Geometry check sheet. Reference: the model listing, model coordinates, mm. A direction names the side the tool comes from. Round coordinates to 2 decimals unless told otherwise and drop trailing zeros. Order: outer loops, then holes, each group sorted by start corner. A loop starts at its lowest first (then second) coordinate and runs counter-clockwise, first axis right, second up. Notation, with made-up numbers: (72, 39) -> (102, 39) arc R27 ccw to (102, 56) -> close; hole circle Ø8 at (86, -27.75). An arc over 180 degrees is marked (long way). Use a Markdown table: item, result. Add a question column.
Item 1: Set-up check for faces 1 (the flat face through (7.875, -18, 1)), 2 (the flat face through (18, -3, 1)), 3 (the flat face through (0, -3, 1)): record each of +Z, -Z, +X, -X, +Y, -Y from which the full face is reachable in a straight line by a thin tool's end or side.
Item 2: Sectioned sample at C-C, the plane x = -3.5. Record the cut outline in (y, z).
Item 3: Sectioned sample at B-B, the plane y = -17. Record the cut outline in (x, z) (3 decimals).
Item 4: Material ranges on probe 1 along X at (y, z) = (-28, 0.75) (3 decimals); probe 2 along Y at (x, z) = (-5, 0.9), recorded low to high. Write a range as [from, to].
Item 5: Sectioned sample at A-A, the plane z = 0.75. Record the cut outline in (x, y) (3 decimals), and give its area (3 significant figures).
Item 6: Gauge pin test, flat end, axial feed: pin 1 Ø0.8 at (y, z) = (-15, 0.5) entering from +X. Record the tip position at first contact, or that the pin passes through.
from build123d import *

# Parameters (mm, degrees)
F1_DEPTH = 1.5


with BuildPart() as f1:
    # F0 (on Top) → F1 (new body)
    with BuildSketch(Plane.XY):
        with BuildLine():
            Line((22.5, 0), (-22.5, 0))
            Line((-22.5, 0), (-22.5, -3))
            Line((-22.5, -3), (-13.5, -3))
            Line((-13.5, -3), (-13.5, -33.25))
            ThreePointArc((-13.5, -33.25), (-13.06066, -34.31066), (-12, -34.75))
            Line((-12, -34.75), (-6.75, -34.75))
            ThreePointArc((-6.75, -34.75), (-5.68934, -34.31066), (-5.25, -33.25))
            Line((-5.25, -33.25), (-5.25, -3))
            Line((-5.25, -3), (5.25, -3))
            Line((5.25, -3), (5.25, -33.25))
            ThreePointArc((5.25, -33.25), (5.68934, -34.31066), (6.75, -34.75))
            Line((6.75, -34.75), (12, -34.75))
            ThreePointArc((12, -34.75), (13.06066, -34.31066), (13.5, -33.25))
            Line((13.5, -33.25), (13.5, -3))
            Line((13.5, -3), (22.5, -3))
            Line((22.5, -3), (22.5, 0))
        make_face()
        with BuildLine():
            ThreePointArc((-10.875, -4.5), (-9.375, -3), (-7.875, -4.5))
            Line((-7.875, -4.5), (-7.875, -30.25))
            ThreePointArc((-7.875, -30.25), (-9.375, -31.75), (-10.875, -30.25))
            Line((-10.875, -30.25), (-10.875, -4.5))
        make_face(mode=Mode.SUBTRACT)
        with BuildLine():
            ThreePointArc((7.875, -4.5), (9.375, -3), (10.875, -4.5))
            Line((10.875, -4.5), (10.875, -30.25))
            ThreePointArc((10.875, -30.25), (9.375, -31.75), (7.875, -30.25))
            Line((7.875, -30.25), (7.875, -4.5))
        make_face(mode=Mode.SUBTRACT)
    extrude(amount=F1_DEPTH)


solid = f1.part
Found:
| question | item | result |
|---|---|---|
| 1 | face 1 | +Z, -Z |
| 1 | face 2 | +Z, -Z, +X, -Y |
| 1 | face 3 | +Z, -Z, -Y |
| 2 | outline | (-3, 0) -> (0, 0) -> (0, 1.5) -> (-3, 1.5) -> close |
| 3 | outline | (-13.5, 0) -> (-10.875, 0) -> (-10.875, 1.5) -> (-13.5, 1.5) -> close; (-7.875, 0) -> (-5.25, 0) -> (-5.25, 1.5) -> (-7.875, 1.5) -> close; (5.25, 0) -> (7.875, 0) -> (7.875, 1.5) -> (5.25, 1.5) -> close; (10.875, 0) -> (13.5, 0) -> (13.5, 1.5) -> (10.875, 1.5) -> close |
| 4 | probe 1 | x = [-13.5, -10.875], [-7.875, -5.25], [5.25, 7.875], [10.875, 13.5] |
| 4 | probe 2 | y = [-3, 0] |
| 5 | outline | (-22.5, -3) -> (-13.5, -3) -> (-13.5, -33.25) arc R1.5 ccw to (-12, -34.75) -> (-6.75, -34.75) arc R1.5 ccw to (-5.25, -33.25) -> (-5.25, -3) -> (5.25, -3) -> (5.25, -33.25) arc R1.5 ccw to (6.75, -34.75) -> (12, -34.75) arc R1.5 ccw to (13.5, -33.25) -> (13.5, -3) -> (22.5, -3) -> (22.5, 0) -> (-22.5, 0) -> close; hole (-10.875, -30.25) arc R1.5 ccw to (-7.875, -30.25) -> (-7.875, -4.5) arc R1.5 ccw to (-10.875, -4.5) -> close; hole (7.875, -30.25) arc R1.5 ccw to (10.875, -30.25) -> (10.875, -4.5) arc R1.5 ccw to (7.875, -4.5) -> close |
| 5 | area | 488 mm2 |
| 6 | pin 1 | stops at x = 13.5 |
